Check sheet for the modelled part. Datum: model origin and axes. Units: mm. A direction names the side the tool comes from. Round coordinates to 2 decimals unless told otherwise and drop trailing zeros. Order: outer loops, then holes, each group sorted by start corner. A loop starts at its lowest first (then second) coordinate and runs counter-clockwise, first axis right, second up. Notation, with made-up numbers: (70.25, -4.75) -> (122.25, -4.75) arc R17 ccw to (122.25, 15.25) -> close; hole circle Ø4 at (-38.75, 71). An arc over 180 degrees is marked (long way). Answer as CSV lines item,"result". Start each with the question number.
Autodesk Fusion 360 part; units mm, degrees
sketch "Esquisse1" plane through (0, 0, 0) normal (0, 0, 1) x (1, 0, 0)
  line L0 (8, 12.5) -> (-8, 12.5)
  line L1 (-8, 12.5) -> (-8, -12.5)
  line L2 (-8, -12.5) -> (8, -12.5)
  line L3 (8, -12.5) -> (8, 12.5)
  line L4 (8, 12.5) -> (-8, -12.5) construction
  line L5 (-8, 12.5) -> (8, -12.5) construction
  dimension "d1" = 16
  dimension "d2" = 25
sketch "Esquisse2" plane through (0, 0, 0) normal (0, 0, 1) x (1, 0, 0)
  line L0 (8, 12.5) -> (-8, 12.5)
  line L1 (-8, 12.5) -> (-8, -12.5)
  line L2 (-8, -12.5) -> (8, -12.5)
  line L3 (8, -12.5) -> (8, 12.5)
  line L4 (8, 12.5) -> (-8, -12.5) construction
  line L5 (-8, 12.5) -> (8, -12.5) construction
  dimension "d5" = 16
  dimension "d6" = 25
extrude "Extrusion2" add sketch "Esquisse2" along normal blind 1
sketch "Esquisse3" plane through (0, 0, 1) normal (0, 0, 1) x (-1, 0, 0)
  line L0 (-8, 12.5) -> (-8, -12.5)
  line L1 (-8, -12.5) -> (8, -12.5)
  line L2 (8, -12.5) -> (8, 12.5)
  line L3 (8, 12.5) -> (-8, 12.5)
  line L4 (-2.475, 3.475) -> (2.475, 3.475)
  line L5 (2.475, 3.475) -> (2.475, -3.475)
  line L6 (2.475, -3.475) -> (-2.475, -3.475)
  line L7 (-2.475, -3.475) -> (-2.475, 3.475)
  line L8 (-2.475, 3.475) -> (2.475, -3.475) construction
  line L9 (2.475, 3.475) -> (-2.475, -3.475) construction
  dimension "d9" = 4.95
  dimension "d10" = 6.95
extrude "Extrusion3" add sketch "Esquisse3" against normal blind 2.49 contours L4 L5 L6 L7
1) Section check A-A on y = 2. Record the cut outline in (x, z) (3 decimals), then the cut area to 3 significant figures.
2) Mould release check, pull along Y, two halves, no side actions. Record for faces 1 (the face through (0, 0, 1)), 2 (the face through (-0.1, -12.5, 0.5)), 3 (the face through (0, 3.475, -1)): released by +Y, released by -Y, zero draft, split by the parting line, or undercut.
3) Depth check by flat-ended pin: pin 1 Ø1.5 at (x, y) = (-1, 4.5) entering from -Z; pin 2 Ø0.7 at (x, z) = (0.5, -1) entering from +Y (3 decimals). Enter the tip coordinate at first touch or a pass-through.
4) Section check C-C on z = -1.15. Record the cut outline in (x, y) (3 decimals), then the cut area to 3 significant figures.
5) Access from +Z, -Z, +X, -X, +Y, -Y to the whole of each face (thin tool, end or side, straight path). Record for faces 4 (the face through (0, -3.475, -1)), 5 (the face through (2.475, 0, -1)), 6 (the face through (-2.475, 0, -1)).
6) Material ranges on line 1 along Z through (x, y) = (5, 6); line 2 along Y through (x, z) = (-0.5, -1.1) (3 decimals); line 3 along X through (y, z) = (-2.25, -1.2) (3 decimals), recorded low to high.
7) Section check B-B on x = -4.75. Record the cut outline in (y, z).
Solutions:
1,outline,"(-8, 0) -> (-2.475, 0) -> (-2.475, -1.49) -> (2.475, -1.49) -> (2.475, 0) -> (8, 0) -> (8, 1) -> (-8, 1) -> close"
1,area,"23.4 mm^2"
2,face 1,"zero draft"
2,face 2,"released by -Y"
2,face 3,"released by +Y"
3,pin 1,"stops at z = 0"
3,pin 2,"stops at y = 3.475"
4,outline,"(-2.475, -3.475) -> (2.475, -3.475) -> (2.475, 3.475) -> (-2.475, 3.475) -> close"
4,area,"34.4 mm^2"
5,face 4,"-Z, +X, -X, -Y"
5,face 5,"-Z, +X, +Y, -Y"
5,face 6,"-Z, -X, +Y, -Y"
6,line 1,"z = 0 to 1"
6,line 2,"y = -3.475 to 3.475"
6,line 3,"x = -2.475 to 2.475"
7,outline,"(-12.5, 0) -> (12.5, 0) -> (12.5, 1) -> (-12.5, 1) -> close"
